```python
from build123d import *

# Parameters (mm, degrees)
F0_W     = 140
F0_H     = 56
F1_DEPTH = 30
F4_D     = 10
F5_D     = 10
F7_DEPTH = 15


with BuildPart() as f1:
    # F0 (on Right) → F1 (new body)
    with BuildSketch(Plane.YZ):
        with Locations((6.608495, -6.87645)):
            Rectangle(F0_W, F0_H)
    extrude(amount=F1_DEPTH)

    # F4 (through all)
    with Locations(Plane.YZ.offset(30)):
        with Locations((-47.391505, -6.87645)):
            Hole(F4_D / 2)

    # F5 (through all)
    with Locations(Plane.YZ.offset(30)):
        with Locations((60.608495, -6.87645)):
            Hole(F5_D / 2)

    # F6 (on Front) → F7 (join)
    with BuildSketch(Plane.XZ):
        Polygon((27.557567, 18.999426), (27.557567, -3.702652), (30.328274, -3.702652), (67.557567, -3.702652), align=None)
        Polygon((30.328274, -3.702652), (27.557567, -3.702652), (27.557567, -33.702652), (67.557567, -33.702652), (67.557567, -3.702652), align=None)
        with BuildLine():
            ThreePointArc((67.557567, -33.702652), (77.557567, -18.702652), (67.557567, -3.702652))
            Line((67.557567, -3.702652), (67.557567, -33.702652))
        make_face()
    extrude(amount=F7_DEPTH)


solid = f1.part
```
CAD build for the part. Positions are in the model's coordinates, mm. A direction names the side the tool comes from. Coordinates: 2 decimals unless noted, no trailing zeros. Order: outer loops, then holes, each group sorted by start corner. A loop starts at its lowest first (then second) coordinate and runs counter-clockwise, first axis right, second up. Notation, with made-up numbers: (35.5, 43) - (76.5, 43) arc R14 ccw to (76.5, 58) - close; hole circle Ø1 at (1, 14). An arc over 180 degrees is marked (long way). Use a Markdown table: item, result. Add a question column.
(1) Which spindle directions (+Z, -Z, +X, -X, +Y, -Y) get a long thin tool onto all of the face, cutting with end or side? Do faces 1 (the face through (49, -7, -33.703)), 2 (the face through (14.79, 64.576, -9.919)). Say none if no direction does.
(2) Flat gauge pins, fed straight in: pin 1 (11.5 mm diameter, centred on y = -47.39, z = -6.88, fed in from +X); pin 2 (7.5 mm diameter, centred on x = 45, y = -7, fed in from -Z); pin 3 (2 mm diameter, centred on x = 51, z = 4, fed in from +Y). Where does each tip first touch, or does it go through?
(3) Drill centre lines: line 1 along Y through (x, z) = (4.5, -5); line 2 along Y through (x, z) = (70.5, -9.5); line 3 along X through (y, z) = (-50, -12). Where is each one in solid material? Low to high. Write a range as [from, to].
(4) Pull direction Y, two halves, no side cores. Call faces 3 (the face through (48, 0, -13)), 4 (the face through (48, -15, -13)), 5 (the face through (14.79, -46.31, -11.76)), 6 (the face through (49.042, -7.395, 6.806)): +Y half, -Y half, draft (parallel to the pull), parting line (faces both ways), or undercut.
(5) Saw through at D-D (x = 62). Give the cut face in (y, z), then the cut area to 3 significant figures.
(6) Saw through at A-A (z = -5.5). Give the cut face in (x, y).
(7) Saw through at B-B (y = 27.5). Give the cut face in (x, z).
(8) Saw through at C-C (z = -16). Give the cut face in (x, y), then the cut area to 3 significant figures.
Solved:
| question | item | result |
|---|---|---|
| 1 | face 1 | -Z, +X, +Y, -Y |
| 1 | face 2 | +X, -X |
| 2 | pin 1 | stops at x = 30 |
| 2 | pin 2 | stops at z = -33.7 |
| 2 | pin 3 | stops at y = 0 |
| 3 | line 1 | y = [-63.39, -52.03], [-42.76, 55.97], [65.24, 76.61] |
| 3 | line 2 | y = [-15, 0] |
| 3 | line 3 | x = [0, 30] |
| 4 | face 3 | +Y half |
| 4 | face 4 | -Y half |
| 4 | face 5 | undercut |
| 4 | face 6 | draft |
| 5 | outline | (-15, -33.7) - (0, -33.7) - (0, -0.55) - (-15, -0.55) - close |
| 5 | area | 497 mm² |
| 6 | outline | (0, -63.39) - (30, -63.39) - (30, -52.2) - (0, -52.2) - close; (0, -42.58) - (30, -42.58) - (30, -15) - (70.78, -15) - (70.78, 0) - (30, 0) - (30, 55.8) - (0, 55.8) - close; (0, 65.42) - (30, 65.42) - (30, 76.61) - (0, 76.61) - close |
| 7 | outline | (0, -34.88) - (30, -34.88) - (30, 21.12) - (0, 21.12) - close |
| 8 | outline | (0, -63.39) - (30, -63.39) - (30, -15) - (77.33, -15) - (77.33, 0) - (30, 0) - (30, 76.61) - (0, 76.61) - close |
| 8 | area | 4,910 mm² |
